```python
from build123d import *

# Parameters (mm, degrees)
SKETCH1_W           = 23.9014
SKETCH1_H           = 21.59
BOSS_EXTRUDE1_DEPTH = 1.27
SKETCH2_W           = 15.621
SKETCH2_H           = 13.462
BOSS_EXTRUDE2_DEPTH = 3.302
SKETCH3_W           = 7.2136
SKETCH3_H           = 7.1628
BOSS_EXTRUDE3_DEPTH = 5.8166
SKETCH4_W           = 4.191
SKETCH4_H           = 7.0358
BOSS_EXTRUDE4_DEPTH = 4.5212
SKETCH5_W           = 4.572
SKETCH5_H           = 9.398
BOSS_EXTRUDE5_DEPTH = 3.81
SKETCH6_W           = 7.874
SKETCH6_H           = 1.961854403
CUT_EXTRUDE1_DEPTH  = 3.81


with BuildPart() as part:
    # Sketch1 → Boss-Extrude1 (new body)
    with BuildSketch(Plane(origin=(0, 0, 0), x_dir=(1, 0, 0), z_dir=(0, 1, 0))):
        with Locations((11.9507, 10.795)):
            Rectangle(SKETCH1_W, SKETCH1_H)
    extrude(amount=BOSS_EXTRUDE1_DEPTH)

    # Sketch2 → Boss-Extrude2 (add)
    with BuildSketch(Plane(origin=(0, 1.27, 0), x_dir=(1, 0, 0), z_dir=(0, 1, 0))):
        with Locations((8.0645, 14.605)):
            Rectangle(SKETCH2_W, SKETCH2_H)
    extrude(amount=BOSS_EXTRUDE2_DEPTH)

    # Sketch3 → Boss-Extrude3 (add)
    with BuildSketch(Plane(origin=(0, 4.572, 0), x_dir=(1, 0, 0), z_dir=(0, 1, 0))):
        with Locations((5.5118, 14.8082)):
            Rectangle(SKETCH3_W, SKETCH3_H)
    extrude(amount=BOSS_EXTRUDE3_DEPTH)

    # Sketch4 → Boss-Extrude4 (add)
    with BuildSketch(Plane(origin=(0, 0, 0), x_dir=(-1, 0, 0), z_dir=(0, -1, 0))):
        with Locations((-10.7569, 13.3477)):
            Rectangle(SKETCH4_W, SKETCH4_H)
    extrude(amount=BOSS_EXTRUDE4_DEPTH)

    # Sketch5 → Boss-Extrude5 (add)
    with BuildSketch(Plane(origin=(0, 0, 0), x_dir=(-1, 0, 0), z_dir=(0, -1, 0))):
        with Locations((-21.3614, 14.4018)):
            Rectangle(SKETCH5_W, SKETCH5_H)
    extrude(amount=BOSS_EXTRUDE5_DEPTH)

    # Sketch6 → Cut-Extrude1 (cut)
    with BuildSketch(Plane(origin=(23.6474, 0, 0), x_dir=(0, 0, -1), z_dir=(1, 0, 0))):
        with Locations((14.4018, -2.067072798)):
            Rectangle(SKETCH6_W, SKETCH6_H)
    extrude(amount=-CUT_EXTRUDE1_DEPTH, mode=Mode.SUBTRACT)


solid = part.part
```
Build history of the part. All positions in model axes, mm. A direction names the side the tool comes from. Round coordinates to 2 decimals unless told otherwise and drop trailing zeros. Loops run counter-clockwise (first coordinate to the right, second up) from the corner with the lowest first, then second, coordinate; pieces in that order, holes last.
Item 1: Saw through at A-A (y = -2). List the corners of the cut face in (x, z), then the cut area to 3 significant figures.
Item 2: Saw through at D-D (x = 12.5). List the corners of the cut face in (y, z), then the cut area to 3 significant figures.
Item 3: Which spindle directions (+Z, -Z, +X, -X, +Y, -Y) get a long thin tool onto all of the face, cutting with end or side? Do faces 1 (the face through (8.661, -2, -13)), 2 (the face through (12.852, -2, -13)), 3 (the face through (15.875, 3, -15)), 4 (the face through (8, 3, -21.336)). Say none if no direction does.
Item 4: Pin check, flat tips, straight feed: P1, Ø10, axis at x = 3, z = -6, coming from the +Y side; P2, Ø1.7, axis at x = 7, y = 6.5, coming from the -Z side; P3, Ø1.9, axis at x = 22, z = -15, coming from the -Y side. Stop position of each tip, or through.
Item 5: Drill centre lines: line 1 along Y through (x, z) = (21.5, -12.75); line 2 along Y through (x, z) = (5.25, -2.5); line 3 along Z through (x, y) = (8.75, 2.25). Where is each one in solid material? Low to high.
Item 6: Saw through at C-C (z = -13). List the corners of the cut face in (x, y) (3 decimals).
Item 7: Saw through at B-B (x = 20.5). List the corners of the cut face in (y, z), then the cut area to 3 significant figures.
Item 8: Two-plate mould, pull along Y, no slides. Class faces 5 (the face through (23.901, 1, -11)), 6 (the face through (21, -3.81, -14)), 7 (the face through (19.837, -2, -14)), 8 (the face through (22, -2, -18.339)): released by +Y, released by -Y, zero draft, split by the parting line, or undercut.
Worked answers:
1. outline: (8.66, -16.87) - (12.85, -16.87) - (12.85, -9.83) - (8.66, -9.83) - close; (19.08, -19.1) - (23.65, -19.1) - (23.65, -18.34) - (19.84, -18.34) - (19.84, -10.46) - (23.65, -10.46) - (23.65, -9.7) - (19.08, -9.7) - close
1. area: 42.5 mm2
2. outline: (-4.52, -16.87) - (0, -16.87) - (0, -21.59) - (1.27, -21.59) - (1.27, -21.34) - (4.57, -21.34) - (4.57, -7.87) - (1.27, -7.87) - (1.27, 0) - (0, 0) - (0, -9.83) - (-4.52, -9.83) - close
2. area: 104 mm2
3. face 1: +Z, -Z, -X, -Y
3. face 2: +Z, -Z, -Y
3. face 3: +Z, -Z, +X, +Y
3. face 4: -Z, +X, -X, +Y
4. P1: stops at y = 4.57
4. P2: stops at z = -18.39
4. P3: stops at y = -3.81
5. line 1: y = -3.81 to -3.05, -1.09 to 1.27
5. line 2: y = 0 to 1.27
5. line 3: z = -21.34 to -7.87
6. outline: (0, 0) - (8.661, 0) - (8.661, -4.521) - (12.852, -4.521) - (12.852, 0) - (19.075, 0) - (19.075, -3.81) - (23.647, -3.81) - (23.647, -3.048) - (19.837, -3.048) - (19.837, -1.086) - (23.647, -1.086) - (23.647, 0) - (23.901, 0) - (23.901, 1.27) - (15.875, 1.27) - (15.875, 4.572) - (9.119, 4.572) - (9.119, 10.389) - (1.905, 10.389) - (1.905, 4.572) - (0.254, 4.572) - (0.254, 1.27) - (0, 1.27) - close
7. outline: (-3.81, -19.1) - (0, -19.1) - (0, -21.59) - (1.27, -21.59) - (1.27, 0) - (0, 0) - (0, -9.7) - (-3.81, -9.7) - close; hole (-3.05, -18.34) - (-1.09, -18.34) - (-1.09, -10.46) - (-3.05, -10.46) - close
7. area: 47.8 mm2
8. face 5: zero draft
8. face 6: released by -Y
8. face 7: undercut
8. face 8: undercut
